```python
from build123d import *

# Parameters (mm, degrees)
PAH1_SIZE             = 0.7
KES_EKSTR_ZYON1_DEPTH = 1.5


with BuildPart() as part:
    # Çizim1 → Döndür1 (revolve)
    with BuildSketch(Plane.XY, mode=Mode.PRIVATE) as d_nd_r1_sk:
        with BuildLine():
            Line((0, 0), (98.3, 0))
            Line((98.3, 0), (98.3, 3))
            Line((98.3, 3), (3.3, 3))
            Line((3.3, 3), (3.3, 5.7))
            Line((3.3, 5.7), (2.6, 5.7))
            ThreePointArc((2.6, 5.7), (0.671107831, 4.848726189), (0, 2.85))
            Line((0, 2.85), (0, 0))
        make_face()
    revolve(d_nd_r1_sk.sketch.rotate(Axis((0, 0, 0), (1, 0, 0)), 180), axis=Axis((0, 0, 0), (1, 0, 0)))

    # Pah1
    pah1_edges = [part.edges().sort_by_distance(p)[0] for p in [
        (98.3, 3, 0),
    ]]
    chamfer(pah1_edges, length=PAH1_SIZE)

    # Çizim2 → Kes-Ekstrüzyon1 (cut)
    with BuildSketch(Plane.ZY):
        Polygon((0, 1.645448267), (-1.425, 0.822724134), (-1.425, -0.822724134), (0, -1.645448267), (1.425, -0.822724134), (1.425, 0.822724134), align=None)
    extrude(amount=-KES_EKSTR_ZYON1_DEPTH, mode=Mode.SUBTRACT)


solid = part.part
```
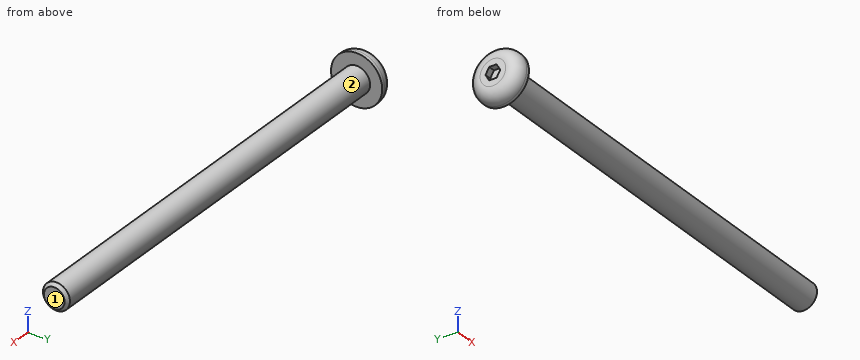
Can you work these out from the model? Positions are in its coordinate system, mm. Face numbers are marked on the shaded views. A direction names the side the tool comes from. Coordinates: 2 decimals unless noted, no trailing zeros. Write each loop counter-clockwise with the first axis right and the second up, starting at its lowest first coordinate (ties: lowest second). Pieces come first, ordered by that corner, then holes. Notation, with made-up numbers: M 63,-28.5 L 96,-28.5 A33 ccw 96,4.5 Z; hole C 41.5,5 d3. An arc over 180 degrees is marked long. Write item = value, one per line. Start each with the question number.
Q1. If I drill on L1, parallel to Z at x = 48, y = -2.5; L2, parallel to X at y = -0.25, z = -2; L3, parallel to X at y = 4, z = -0.75, over which ranges is the centre line in solid material (lowest first)? Write a range as [from, to].
Q2. On a 3-axis mill with a long thin cutter (end or side, diameter ignored), from which of +Z, -Z, +X, -X, +Y, -Y can I reach the whole of each face in a straight line? I mean the marked faces 1 and 2. Say none if no direction works.
Q3. I'm going to push flat-ended pins straight in: pin 1 (1.2 mm diameter, centred on x = 1, y = 0.5, fed in from -Z); pin 2 (1 mm diameter, centred on x = 70.5, z = -3, fed in from -Y); pin 3 (3 mm diameter, centred on y = -0.5, z = -1, fed in from -X). Where does each tip first touch, or does it pass through?
Q4. If we section it at A-A, the plane y = 0: Write out the boundary of the cut face in (x, z) (3 decimals).
Q5. If we section it at B-B, the plane x = 11.5: Write out the boundary of the cut face in (y, z).
Check sheet entries:
q1.L1 = [-1.66, 1.66]
q1.L2 = [0, 98.3]
q1.L3 = [0.18, 3.3]
q2.face_1 = +Z, -Z, +X, +Y, -Y
q2.face_2 = +X
q3.pin_1 = -5.48
q3.pin_2 = -1.66
q3.pin_3 = 0
q4.outline = M 0,-2.85 A2.611 ccw 2.6,-5.7 L 3.3,-5.7 L 3.3,-3 L 97.6,-3 L 98.3,-2.3 L 98.3,2.3 L 97.6,3 L 3.3,3 L 3.3,5.7 L 2.6,5.7 A2.611 ccw 0,2.85 L 0,1.425 L 1.5,1.425 L 1.5,-1.425 L 0,-1.425 Z
q5.outline = C 0,0 d6
